Design review of the part built by this model. Coordinates are the model's own, in mm. Give positions to 0.01 mm unless a question says otherwise; leave off trailing zeros. Write each loop counter-clockwise with the first axis right and the second up, starting at its lowest first coordinate (ties: lowest second). Pieces come first, ordered by that corner, then holes. Notation, with made-up numbers: M 1.25,21.25 L 17.25,21.25 A31 ccw 17.25,57.25 Z; hole C -18,57 d4. An arc over 180 degrees is marked long. Answer in a Markdown table with one row per item.
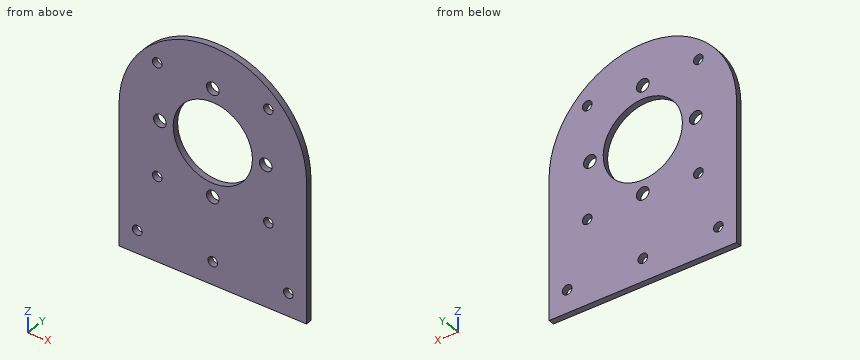
```python
from build123d import *

# Parameters (mm, degrees)
SKETCH_1_R      = 1.6
SKETCH_1_R_2    = 31
SKETCH_1_R_3    = 21
SKETCH_1_R_4    = 2.1
SKETCH_1_R_5    = 13.1
EXTRUDE_1_DEPTH = 2


with BuildPart() as part:
    # 草图1 → 凸台-拉伸1 (new body)
    # profile 1 of 3: a face of its own
    with BuildSketch(Plane(origin=(0, 0, 0), x_dir=(1, 0, 0), z_dir=(0, 1, 0))):
        with BuildLine():
            Line((-31, 31), (-31, 0))
            ThreePointArc((-31, 0), (0, 31), (31, 0))
            Line((31, 0), (31, 31))
            Line((31, 31), (31, 46))
            Line((31, 46), (-31, 46))
            Line((-31, 46), (-31, 31))
        make_face()
        with Locations(Location((-25, 38.5, 0), (0, 0, 270))):
            Circle(SKETCH_1_R, mode=Mode.SUBTRACT)
        with Locations(Location((0, 38.5, 0), (0, 0, 270))):
            Circle(SKETCH_1_R, mode=Mode.SUBTRACT)
        with Locations(Location((25, 38.5, 0), (0, 0, 270))):
            Circle(SKETCH_1_R, mode=Mode.SUBTRACT)
    # profile 2 of 3: a face of its own
    with BuildSketch(Plane(origin=(0, 0, 0), x_dir=(1, 0, 0), z_dir=(0, 1, 0))):
        Circle(SKETCH_1_R_2)
        with Locations(Location((-18.384776311, 18.384776311, 0), (0, 0, 270))):
            Circle(SKETCH_1_R, mode=Mode.SUBTRACT)
        with Locations(Location((-18.384776311, -18.384776311, 0), (0, 0, 270))):
            Circle(SKETCH_1_R, mode=Mode.SUBTRACT)
        with Locations(Location((18.384776311, -18.384776311, 0), (0, 0, 270))):
            Circle(SKETCH_1_R, mode=Mode.SUBTRACT)
        with Locations(Location((18.384776311, 18.384776311, 0), (0, 0, 270))):
            Circle(SKETCH_1_R, mode=Mode.SUBTRACT)
        Circle(SKETCH_1_R_3, mode=Mode.SUBTRACT)
    # profile 3 of 3: a face of its own
    with BuildSketch(Plane(origin=(0, 0, 0), x_dir=(1, 0, 0), z_dir=(0, 1, 0))):
        Circle(SKETCH_1_R_3)
        with Locations(Location((17.5, 0, 0), (0, 0, 270))):
            Circle(SKETCH_1_R_4, mode=Mode.SUBTRACT)
        with Locations(Location((0, -17.5, 0), (0, 0, 270))):
            Circle(SKETCH_1_R_4, mode=Mode.SUBTRACT)
        with Locations(Location((-17.5, 0, 0), (0, 0, 270))):
            Circle(SKETCH_1_R_4, mode=Mode.SUBTRACT)
        with Locations(Location((0, 17.5, 0), (0, 0, 270))):
            Circle(SKETCH_1_R_4, mode=Mode.SUBTRACT)
        with Locations(Location((0, 0, 0), (0, 0, 270))):
            Circle(SKETCH_1_R_5, mode=Mode.SUBTRACT)
    extrude(amount=EXTRUDE_1_DEPTH)


solid = part.part
```
1) To check wall thickness, follow probe 1 along X at (y, z) = (0.4, 0); probe 2 along X at (y, z) = (0.85, -38.5); probe 3 along Z at (x, y) = (-18, 1.5). State the ranges of each line that lie inside material, in increasing order. Write a range as [from, to].
Geometry says:
| item | result |
|---|---|
| probe 1 | [-31, -19.6], [-15.4, -13.1], [13.1, 15.4], [19.6, 31] |
| probe 2 | [-31, -26.6], [-23.4, -1.6], [1.6, 23.4], [26.6, 31] |
| probe 3 | [-46, -19.94], [-16.83, -2.04], [2.04, 16.83], [19.94, 25.24] |
2) Add section B-B (z = -3). Write out the cut boundary in (x, y).
Geometry says:
| item | result |
|---|---|
| outline | M -31,0 L -12.75,0 L -12.75,2 L -31,2 Z; M 12.75,0 L 31,0 L 31,2 L 12.75,2 Z |
3) Add section A-A (x = 0). Write out the cut boundary in (y, z).
Geometry says:
| item | result |
|---|---|
| outline | M 0,-46 L 2,-46 L 2,-40.1 L 0,-40.1 Z; M 0,-36.9 L 2,-36.9 L 2,-19.6 L 0,-19.6 Z; M 0,-15.4 L 2,-15.4 L 2,-13.1 L 0,-13.1 Z; M 0,13.1 L 2,13.1 L 2,15.4 L 0,15.4 Z; M 0,19.6 L 2,19.6 L 2,31 L 0,31 Z |
4) Add section D-D (y = 1.65). Count the separate pieces of the cut face and the enclosed holes in it, and give its area (3 significant figures).
Geometry says:
| item | result |
|---|---|
| separate pieces | 1 |
| enclosed holes | 12 |
| area | 3,710 mm^2 |
5) Add section C-C (x = -25). Write out the cut boundary in (y, z), and give its area (3 significant figures).
Geometry says:
| item | result |
|---|---|
| outline | M 0,-46 L 2,-46 L 2,-40.1 L 0,-40.1 Z; M 0,-36.9 L 2,-36.9 L 2,18.33 L 0,18.33 Z |
| area | 122 mm^2 |
